Work out the finished part from the listing and answer in its coordinate system (mm). Face numbers are marked on the shaded views. A direction names the side the tool comes from. Give positions to 0.01 mm unless a question says otherwise; leave off trailing zeros. Loops run counter-clockwise (first coordinate to the right, second up) from the corner with the lowest first, then second, coordinate; pieces in that order, holes last. Notation, with made-up numbers: (11.25, -35) - (55.25, -35) arc R10 cw to (55.25, -20) - close; hole circle Ø8 at (44.5, 2). An arc over 180 degrees is marked (long way). One line per question, with ' | ' between items.
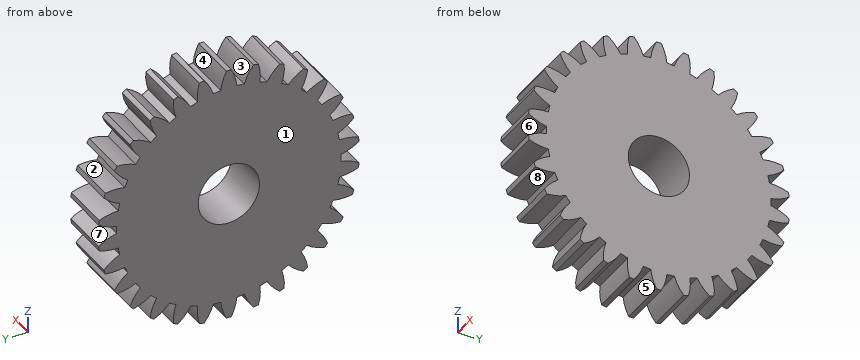
from build123d import *

# Parameters (mm, degrees)
BASPROSKE_W     = 12
BASPROSKE_H     = 32
TOOTHCUT_DEPTH  = 13
TEETHCUTS_COUNT = 30
TEETHCUTS_ANGLE = 348
BORSKE_R        = 7.5
BORE_DEPTH      = 50.0000508


with BuildPart() as part:
    # BasProSke → Base-Revolve (revolve)
    with BuildSketch(Plane(origin=(0, 0, 0), x_dir=(1, 0, 0), z_dir=(0, 1, 0))):
        with Locations((6, 16)):
            Rectangle(BASPROSKE_W, BASPROSKE_H)
    revolve(axis=Axis((-10, 0, 0), (1, 0, 0)))

    # TooCutSke → ToothCut (cut, through all)
    with BuildSketch(Plane(origin=(0, 0, 0), x_dir=(0, 0, -1), z_dir=(1, 0, 0))):
        with BuildLine():
            ThreePointArc((0.918551563, 27.483654488), (0, 27.499), (-0.918551563, 27.483654488))
            ThreePointArc((-0.918551563, 27.483654488), (-1.617208176, 29.787801627), (-2.761784709, 31.906093311))
            ThreePointArc((-2.761784709, 31.906093311), (0, 32.0254), (2.761784709, 31.906093311))
            ThreePointArc((2.761784709, 31.906093311), (1.617208176, 29.787801627), (0.918551563, 27.483654488))
        make_face()
    toothcut = extrude(amount=TOOTHCUT_DEPTH, mode=Mode.SUBTRACT)

    # TeethCuts: ToothCut ×30 about axis
    teethcuts_axis = Axis((-10, 0, 0), (1, 0, 0))
    for i in range(1, TEETHCUTS_COUNT):
        add(toothcut.rotate(teethcuts_axis, i * TEETHCUTS_ANGLE / (TEETHCUTS_COUNT - 1)), mode=Mode.SUBTRACT)

    # BorSke → Bore (cut, symmetric)
    with BuildSketch(Plane(origin=(0, 0, 0), x_dir=(0, 0, -1), z_dir=(1, 0, 0))):
        Circle(BORSKE_R)
    extrude(amount=BORE_DEPTH, both=True, mode=Mode.SUBTRACT)


solid = part.part
1. Flat-ended cylindrical pins translate along their axes: pin 1 (1 mm diameter, centred on x = 4.5, y = 20, fed in from -Z); pin 2 (4 mm diameter, centred on x = 10.5, z = 13.5, fed in from +Y); pin 3 (1.5 mm diameter, centred on x = 3, z = -7.5, fed in from +Y). Find the tip coordinate at first contact, or state that the pin passes through.
Evaluation:
pin 1: z = -20.73 | pin 2: y = 28.01 | pin 3: y = 29.44
2. Determine the mould class of the marked faces 1, 2 and 3 for opening direction Z: +Z half, -Z half, draft (parallel to the pull), parting line (faces both ways), or undercut.
Evaluation:
face 1: draft | face 2: undercut | face 3: +Z half
3. Find section A-A on z = 0. Write down the section's boundary in (x, y).
Evaluation:
outline: (0, -27.5) - (12, -27.5) - (12, -7.5) - (0, -7.5) - close; (0, 7.5) - (12, 7.5) - (12, 27.5) - (0, 27.5) - close
4. Find section B-B on z = 18. Write down the section's boundary in (x, y).
Evaluation:
outline: (0, -22.6) - (12, -22.6) - (12, 22.6) - (0, 22.6) - close
5. Consider L1, parallel to Y at x = 8.25, z = 0; L2, parallel to Y at x = 6.25, z = -28.5; L3, parallel to Y at x = 4.75, z = -20. Determine where each line is inside the solid, lowest interval first.
Evaluation:
L1: -27.5 to -7.5, 7.5 to 27.5 | L2: -13.59 to -11.36, -7.69 to -4.25, -1.81 to 1.81, 4.25 to 7.69, 11.36 to 13.59 | L3: -23.78 to -19.33, -18.87 to 18.87, 19.33 to 23.78
6. Which of the six approach directions +Z, -Z, +X, -X, +Y, -Y give full straight-line access (tool end or side, diameter ignored) to the marked faces 4, 5, 6, 7 and 8?
Evaluation:
face 4: +Z, +X, -X | face 5: -Z, +X, -X | face 6: +X, -X, -Y | face 7: +X, -X, +Y | face 8: +X, -X
